Geometry: final body of the model. Coordinates: model frame, mm. A direction names the side the tool comes from. Give positions to 0.01 mm unless a question says otherwise; leave off trailing zeros. Order: outer loops, then holes, each group sorted by start corner. A loop starts at its lowest first (then second) coordinate and runs counter-clockwise, first axis right, second up. Notation, with made-up numbers: (14.25, 20) - (38.25, 20) arc R17 cw to (38.25, 52) - close; hole circle Ø7 at (78.5, -25). An arc over 180 degrees is marked (long way). Use one line per item in the form item = value.
from build123d import *

# Parameters (mm, degrees)
SKETCH1_R           = 1.5
SKETCH1_W           = 20
SKETCH1_H           = 3.2
BOSS_EXTRUDE1_DEPTH = 3


with BuildPart() as part:
    # Sketch1 → Boss-Extrude1 (new body)
    with BuildSketch(Plane.XY):
        with BuildLine():
            Line((10, 120), (10, 123))
            Line((10, 123), (-10, 123))
            Line((-10, 123), (-10, 120))
            Line((-10, 120), (-13.265006005, 120))
            ThreePointArc((-13.265006005, 120), (-32, 111), (-50.734993995, 120))
            Line((-50.734993995, 120), (-55, 120))
            ThreePointArc((-55, 120), (-57.121320344, 119.121320344), (-58, 117))
            Line((-58, 117), (-58, 114))
            Line((-58, 114), (-68, 114))
            ThreePointArc((-68, 114), (-67.006266357, 91.089484919), (-58, 70))
            Line((-58, 70), (-58, 20))
            Line((-58, 20), (-61, 20))
            Line((-61, 20), (-61, 0))
            Line((-61, 0), (-58, 0))
            Line((-58, 0), (-58, -60))
            Line((-58, -60), (58, -60))
            Line((58, -60), (58, 0))
            Line((58, 0), (61, 0))
            Line((61, 0), (61, 20))
            Line((61, 20), (58, 20))
            Line((58, 20), (58, 70))
            ThreePointArc((58, 70), (67.006266357, 91.089484919), (68, 114))
            Line((68, 114), (58, 114))
            Line((58, 114), (58, 117))
            ThreePointArc((58, 117), (57.121320344, 119.121320344), (55, 120))
            Line((55, 120), (50.734993995, 120))
            ThreePointArc((50.734993995, 120), (32, 111), (13.265006005, 120))
            Line((13.265006005, 120), (10, 120))
        make_face()
        with Locations((-55, 99)):
            Circle(SKETCH1_R, mode=Mode.SUBTRACT)
        with Locations((-30.94, 99)):
            Circle(SKETCH1_R, mode=Mode.SUBTRACT)
        with Locations((-55, 69.11)):
            Circle(SKETCH1_R, mode=Mode.SUBTRACT)
        with Locations((-30.94, 69.11)):
            Circle(SKETCH1_R, mode=Mode.SUBTRACT)
        with Locations((30.94, 99)):
            Circle(SKETCH1_R, mode=Mode.SUBTRACT)
        with Locations((55, 99)):
            Circle(SKETCH1_R, mode=Mode.SUBTRACT)
        with Locations((30.94, 69.11)):
            Circle(SKETCH1_R, mode=Mode.SUBTRACT)
        with Locations((55, 69.11)):
            Circle(SKETCH1_R, mode=Mode.SUBTRACT)
        with Locations((-50, -36.5)):
            Circle(SKETCH1_R, mode=Mode.SUBTRACT)
        with Locations((50, -36.5)):
            Circle(SKETCH1_R, mode=Mode.SUBTRACT)
        with Locations((-12.5, 115)):
            Circle(SKETCH1_R, mode=Mode.SUBTRACT)
        with Locations((12.5, 115)):
            Circle(SKETCH1_R, mode=Mode.SUBTRACT)
        with Locations((-43.75, 108)):
            Circle(SKETCH1_R, mode=Mode.SUBTRACT)
        with Locations((43.75, 108)):
            Circle(SKETCH1_R, mode=Mode.SUBTRACT)
        with Locations((-43.75, -7.5)):
            Circle(SKETCH1_R, mode=Mode.SUBTRACT)
        with Locations((43.75, -7.5)):
            Circle(SKETCH1_R, mode=Mode.SUBTRACT)
        with Locations((-52, 24)):
            Circle(SKETCH1_R, mode=Mode.SUBTRACT)
        with Locations((52, 24)):
            Circle(SKETCH1_R, mode=Mode.SUBTRACT)
        with Locations((-52, 115)):
            Circle(SKETCH1_R, mode=Mode.SUBTRACT)
        with Locations((52, 115)):
            Circle(SKETCH1_R, mode=Mode.SUBTRACT)
        with Locations((0, 61.6)):
            Rectangle(SKETCH1_W, SKETCH1_H, mode=Mode.SUBTRACT)
        with BuildLine():
            Line((-48, 60.5), (-48, 35.5))
            ThreePointArc((-48, 35.5), (-51, 32.5), (-54, 35.5))
            Line((-54, 35.5), (-54, 60.5))
            ThreePointArc((-54, 60.5), (-51, 63.5), (-48, 60.5))
        make_face(mode=Mode.SUBTRACT)
        with BuildLine():
            Line((54, 60.5), (54, 35.5))
            ThreePointArc((54, 35.5), (51, 32.5), (48, 35.5))
            Line((48, 35.5), (48, 60.5))
            ThreePointArc((48, 60.5), (51, 63.5), (54, 60.5))
        make_face(mode=Mode.SUBTRACT)
        with BuildLine():
            Line((-48, 5.5), (-48, -19.5))
            ThreePointArc((-48, -19.5), (-51, -22.5), (-54, -19.5))
            Line((-54, -19.5), (-54, 5.5))
            ThreePointArc((-54, 5.5), (-51, 8.5), (-48, 5.5))
        make_face(mode=Mode.SUBTRACT)
        with BuildLine():
            Line((54, 5.5), (54, -19.5))
            ThreePointArc((54, -19.5), (51, -22.5), (48, -19.5))
            Line((48, -19.5), (48, 5.5))
            ThreePointArc((48, 5.5), (51, 8.5), (54, 5.5))
        make_face(mode=Mode.SUBTRACT)
        with BuildLine():
            Line((-12.5, -21), (12.5, -21))
            ThreePointArc((12.5, -21), (17.5, -26), (12.5, -31))
            Line((12.5, -31), (-12.5, -31))
            ThreePointArc((-12.5, -31), (-17.5, -26), (-12.5, -21))
        make_face(mode=Mode.SUBTRACT)
    extrude(amount=BOSS_EXTRUDE1_DEPTH)


solid = part.part
(1) Reachability of faces 4 (the face through (-17.5, -26.1, 1.5)), 5 (the face through (-67.077, 91.404, 1.479)) from +Z, -Z, +X, -X, +Y, -Y: full face, straight path, thin tool, end or side. Return the list, or none.
Computed values:
face_4 = +Z, -Z
face_5 = +Z, -Z, -X
(2) Cut plane C-C on z = 1.7. Give the number of separate pieces and of enclosed holes in the cut face, plus the area to 3 significant figures.
Computed values:
separate_pieces = 1
enclosed_holes = 26
area = 20,000 mm²
(3) Cut plane B-B on y = 40. Output: boundary loops of the cut face in (x, z), plus the area to 3 significant figures.
Computed values:
outline = (-58, 0) - (-54, 0) - (-54, 3) - (-58, 3) - close; (-48, 0) - (48, 0) - (48, 3) - (-48, 3) - close; (54, 0) - (58, 0) - (58, 3) - (54, 3) - close
area = 312 mm²
(4) Cut plane D-D on y = -45.5. Output: boundary loops of the cut face in (x, z), plus the area to 3 significant figures.
Computed values:
outline = (-58, 0) - (58, 0) - (58, 3) - (-58, 3) - close
area = 348 mm²
(5) Ray query, line 1 along Y through (x, z) = (-12.5, 1); line 2 along X through (y, z) = (69.11, 1.15); line 3 along Y through (x, z) = (-6.5, 1.2). Return the intervals inside material, ascending.
Computed values:
line_1 = -60 to -31, -21 to 113.5, 116.5 to 120
line_2 = -58 to -56.5, -53.5 to -32.44, -29.44 to 29.44, 32.44 to 53.5, 56.5 to 58
line_3 = -60 to -31, -21 to 60, 63.2 to 123
(6) Pull-direction query (Y, two-part tool) for faces 1 (the face through (-1, 33, 0)), 2 (the face through (17.5, -25.9, 1.5)), 3 (the face through (32, 111, 1)); classes: released by +Y, released by -Y, zero draft, split by the parting line, or undercut.
Computed values:
face_1 = zero draft
face_2 = undercut
face_3 = released by +Y
(7) Contact query for flat-ended pins moving along their axis: pin 1 Ø1.5 at (x, z) = (-60, 1.5) entering from -Y; pin 2 Ø1 at (x, z) = (33, 1.5) entering from +Y; pin 3 Ø1.5 at (x, z) = (-59, 2) entering from +Y. Output: stop coordinate, or through.
Computed values:
pin_1 = 0
pin_2 = 111.05
pin_3 = 114
(8) Cut plane A-A on y = -26. Output: boundary loops of the cut face in (x, z).
Computed values:
outline = (-58, 0) - (-17.5, 0) - (-17.5, 3) - (-58, 3) - close; (17.5, 0) - (58, 0) - (58, 3) - (17.5, 3) - close
